Can you work these out from the model? Positions are in its coordinate system, mm. A direction names the side the tool comes from. Give positions to 0.01 mm unless a question says otherwise; leave off trailing zeros. Write each loop counter-clockwise with the first axis right and the second up, starting at its lowest first coordinate (ties: lowest second). Pieces come first, ordered by that corner, then holes.
```python
from build123d import *

# Parameters (mm, degrees)
SKETCH_1_W           = 46
SKETCH_1_H           = 20
EXTRUDE_1_DEPTH      = 4
SKETCH_2_R           = 8.25
CUT_EXTRUDE_1_DEPTH  = 5
SKETCH_3_W           = 8
SKETCH_3_H           = 6
CUT_EXTRUDE_2_DEPTH  = 5
SKETCH_4_W           = 5
SKETCH_4_H           = 4
CUT_EXTRUDE_3_DEPTH  = 5
SKETCH_5_W           = 3
SKETCH_5_H           = 2
SKETCH_5_W_2         = 2
SKETCH_5_H_2         = 3
CUT_EXTRUDE_4_DEPTH  = 1
SKETCH_6_W           = 46
SKETCH_6_H           = 4
EXTRUDE_2_DEPTH      = 22.5
SKETCH_8_W           = 15
SKETCH_8_H           = 3.5
EXTRUDE_4_DEPTH      = 46
CHAMFER_3_SIZE       = 5
SKETCH_9_R           = 2.1
CUT_EXTRUDE_5_DEPTH  = 4.5
SKETCH_10_R          = 2.1
CUT_EXTRUDE_6_DEPTH  = 20
SKETCH_13_W          = 10
SKETCH_13_H          = 8
CUT_EXTRUDE_9_DEPTH  = 46
SKETCH_14_R          = 1.6
CUT_EXTRUDE_10_DEPTH = 46


with BuildPart() as part:
    # 草圖1 → 填料-伸長1 (new body)
    with BuildSketch(Plane.XY):
        Rectangle(SKETCH_1_W, SKETCH_1_H)
    extrude(amount=EXTRUDE_1_DEPTH)

    # 草圖2 → 除料-伸長1 (cut, through all)
    with BuildSketch(Plane.XY.offset(4)):
        with Locations((-12.7, -0.65)):
            Circle(SKETCH_2_R)
        with Locations((12.7, -0.65)):
            Circle(SKETCH_2_R)
    extrude(amount=-CUT_EXTRUDE_1_DEPTH, mode=Mode.SUBTRACT)

    # 草圖3 → 除料-伸長2 (cut, through all)
    with BuildSketch(Plane.XY.offset(4)):
        with Locations((0, 7)):
            Rectangle(SKETCH_3_W, SKETCH_3_H)
    extrude(amount=-CUT_EXTRUDE_2_DEPTH, mode=Mode.SUBTRACT)

    # 草圖4 → 除料-伸長3 (cut, through all)
    with BuildSketch(Plane.XY.offset(4)):
        with Locations((0, -5.5)):
            Rectangle(SKETCH_4_W, SKETCH_4_H)
    extrude(amount=-CUT_EXTRUDE_3_DEPTH, mode=Mode.SUBTRACT)

    # 草圖5 → 除料-伸長4 (cut)
    with BuildSketch(Plane.XY.offset(4)):
        with Locations((4, -6.5)):
            Rectangle(SKETCH_5_W, SKETCH_5_H)
        with Locations((-5.5, 8)):
            Rectangle(SKETCH_5_W_2, SKETCH_5_H_2)
        with Locations((5.5, 8)):
            Rectangle(SKETCH_5_W_2, SKETCH_5_H_2)
    extrude(amount=-CUT_EXTRUDE_4_DEPTH, mode=Mode.SUBTRACT)

    # 草圖6 → 填料-伸長2 (add)
    with BuildSketch(Plane.XZ.offset(10)):
        with Locations((0, 2)):
            Rectangle(SKETCH_6_W, SKETCH_6_H)
    extrude(amount=EXTRUDE_2_DEPTH)

    # 草圖8 → 填料-伸長4 (add)
    with BuildSketch(Plane.ZY.offset(23)):
        with Locations((11.5, -30.75)):
            Rectangle(SKETCH_8_W, SKETCH_8_H)
    extrude(amount=-EXTRUDE_4_DEPTH)

    # 導角3
    chamfer_3_edges = [part.edges().sort_by_distance(p)[0] for p in [
        (0, -29, 4),
        (0, -32.5, 0),
    ]]
    chamfer(chamfer_3_edges, length=CHAMFER_3_SIZE)

    # 草圖9 → 除料-伸長5 (cut, through all)
    with BuildSketch(Plane(origin=(0, -29, 0), x_dir=(1, 0, 0), z_dir=(0, 1, 0))):
        with Locations((0, -12)):
            Circle(SKETCH_9_R)
    extrude(amount=-CUT_EXTRUDE_5_DEPTH, mode=Mode.SUBTRACT)

    # 草圖10 → 除料-伸長6 (cut, through all)
    with BuildSketch(Plane(origin=(0, 0, 0), x_dir=(-1, 0, 0), z_dir=(0, 0, -1))):
        with Locations((0, -25)):
            Circle(SKETCH_10_R)
    extrude(amount=-CUT_EXTRUDE_6_DEPTH, mode=Mode.SUBTRACT)

    # 草圖13 → 除料-伸長9 (cut)
    with BuildSketch(Plane.XY.offset(4)):
        with Locations((0, -25)):
            Rectangle(SKETCH_13_W, SKETCH_13_H)
    extrude(amount=CUT_EXTRUDE_9_DEPTH, mode=Mode.SUBTRACT)

    # 草圖14 → 除料-伸長10 (cut)
    with BuildSketch(Plane.XY.offset(4)):
        with Locations((-21, 8)):
            Circle(SKETCH_14_R)
    extrude(amount=-CUT_EXTRUDE_10_DEPTH, mode=Mode.SUBTRACT)


solid = part.part
```
1) Suppose I cut it at D-D on x = 0. Write out the boundary of the cut face in (y, z).
Values follow:
outline: (-32.5, 5) - (-27.5, 0) - (-27.1, 0) - (-27.1, 4) - (-29, 4) - (-29, 9.9) - (-32.5, 9.9) - close; (-32.5, 14.1) - (-29, 14.1) - (-29, 19) - (-32.5, 19) - close; (-22.9, 0) - (-7.5, 0) - (-7.5, 4) - (-22.9, 4) - close; (-3.5, 0) - (4, 0) - (4, 4) - (-3.5, 4) - close
2) For faces 1 (the face through (2.5, -6, 2)), 2 (the face through (-4, 7, 2)), 3 (the face through (-5.5, 9.5, 3.5)), which set-ups out of +Z, -Z, +X, -X, +Y, -Y let a thin tool reach every point of the face, with its end or its side?
Values follow:
face 1: +Z, -Z
face 2: +Z, -Z, +Y
face 3: +Z
3) If we mould it in two halves opening along X, with no side actions, what happens to faces 4 (the face through (5.5, 6.5, 3.5)), 5 (the face through (13, 10, 2))? For each: +X half, -X half, draft (parallel to the pull), parting line (faces both ways), or undercut.
Values follow:
face 4: undercut
face 5: draft
4) Suppose I cut it at A-A on x = -12.7. Write out the boundary of the cut face in (y, z).
Values follow:
outline: (-32.5, 5) - (-27.5, 0) - (-8.9, 0) - (-8.9, 4) - (-24, 4) - (-29, 9) - (-29, 19) - (-32.5, 19) - close; (7.6, 0) - (10, 0) - (10, 4) - (7.6, 4) - close
5) Suppose I cut it at C-C on y = -25. Write out the boundary of the cut face in (x, z).
Values follow:
outline: (-23, 0) - (-2.1, 0) - (-2.1, 4) - (-5, 4) - (-5, 5) - (-23, 5) - close; (2.1, 0) - (23, 0) - (23, 5) - (5, 5) - (5, 4) - (2.1, 4) - close
6) For pin 1 Ø5 at (x, y) = (0, -25) entering from +Z; pin 2 Ø4.5 at (x, z) = (11, 8.5) entering from +Y; pin 3 Ø1.2 at (x, z) = (-1, 1.5) entering from +Y, each with a flat end and sliding along its axis, tell me the tip position at first contact or that it passes through.
Values follow:
pin 1: stops at z = 4
pin 2: stops at y = -26.25
pin 3: stops at y = 4
7) Please list where these lines run through material, in increasing order: L1, parallel to X at y = -31.45, z = 12; L2, parallel to X at y = -28, z = 6.5; L3, parallel to Z at x = -4, y = -15.
Values follow:
L1: x = -23 to -2.1, 2.1 to 23
L2: x = -23 to -5, 5 to 23
L3: z = 0 to 4
8) Suppose I cut it at B-B on z = 12. Write out the boundary of the cut face in (x, y).
Values follow:
outline: (-23, -32.5) - (-2.1, -32.5) - (-2.1, -29) - (-23, -29) - close; (2.1, -32.5) - (23, -32.5) - (23, -29) - (2.1, -29) - close
